from build123d import *

# Parameters (mm, degrees)
BOSS_EXTRUDE1_DEPTH = 12.7
SKETCH2_W           = 330.2
SKETCH2_H           = 19.05
CUT_EXTRUDE1_DEPTH  = 13.7
SKETCH3_R           = 1.27
CUT_EXTRUDE2_DEPTH  = 356.6
CUT_EXTRUDE7_DEPTH  = 6.35


with BuildPart() as part:
    # Sketch1 → Boss-Extrude1 (new body)
    with BuildSketch(Plane.XY):
        Polygon((0, 0), (355.6, 0), (355.6, -223.774), (274.574, -304.751813258), (81.026, -304.751813258), (0, -223.774), align=None)
    extrude(amount=BOSS_EXTRUDE1_DEPTH)

    # Sketch2 → Cut-Extrude1 (cut, through all)
    with BuildSketch(Plane.XY.offset(12.7)):
        with Locations((177.8, -9.525)):
            Rectangle(SKETCH2_W, SKETCH2_H)
    extrude(amount=-CUT_EXTRUDE1_DEPTH, mode=Mode.SUBTRACT)

    # Sketch3 → Cut-Extrude2 (cut, through all)
    with BuildSketch(Plane.ZY):
        with Locations((6.35, -6.35)):
            Circle(SKETCH3_R)
    extrude(amount=-CUT_EXTRUDE2_DEPTH, mode=Mode.SUBTRACT)

    # Sketch4 → Cut-Extrude7 (cut)
    with BuildSketch(Plane.XY):
        Polygon((10.3378, -45.974), (10.3378, -219.490141692), (85.306255844, -294.414013258), (86.209906071, -292.23149061), (12.520322648, -218.58573091), (12.520322648, -45.974), align=None)
        Polygon((270.293744156, -294.414013258), (345.2622, -219.490141692), (345.2622, -45.974), (342.9, -45.974), (342.9, -218.511274805), (269.416328936, -292.294854171), align=None)
    extrude(amount=CUT_EXTRUDE7_DEPTH, mode=Mode.SUBTRACT)


solid = part.part
Part model, mm, in its own coordinate system. A direction names the side the tool comes from. Give positions to 0.01 mm unless a question says otherwise; leave off trailing zeros. Write each loop counter-clockwise with the first axis right and the second up, starting at its lowest first coordinate (ties: lowest second). Pieces come first, ordered by that corner, then holes.
1) Probe L1, parallel to X at y = -201, z = 5.25; L2, parallel to Z at x = 2, y = -6; L3, parallel to X at y = -12, z = 5.25. List the from-to ranges inside material, lowest first.
Resolved:
L1: x = 0 to 10.34, 12.52 to 342.9, 345.26 to 355.6
L2: z = 0 to 5.13, 7.57 to 12.7
L3: x = 0 to 12.7, 342.9 to 355.6
2) Cut at A-A on z = 10.25. Write the cut outline in (x, y), then the cut area to 3 significant figures.
Resolved:
outline: (0, -223.77) - (81.03, -304.75) - (274.57, -304.75) - (355.6, -223.77) - (355.6, 0) - (342.9, 0) - (342.9, -19.05) - (12.7, -19.05) - (12.7, 0) - (0, 0) - close
area: 95,500 mm2
3) Pin check, flat tips, straight feed: pin 1 (2 mm diameter, centred on x = 43, z = 2, fed in from -Y); pin 2 (3 mm diameter, centred on x = 309.5, z = 3.5, fed in from -Y); pin 3 (3 mm diameter, centred on y = -6.35, z = 6.35, fed in from +X); pin 4 (2 mm diameter, centred on x = 235, z = 10.5, fed in from +Y). Stop position of each tip, or through.
Resolved:
pin 1: stops at y = -267.75
pin 2: stops at y = -271.35
pin 3: stops at x = 355.6
pin 4: stops at y = -19.05
4) Two-plate mould, pull along X, no slides. Class faces 1 (the face through (175, -19.05, 6)), 2 (the face through (179, -304.752, 6)), 3 (the face through (0, -113, 6)), 4 (the face through (315.65, -263.7, 6.26)): released by +X, released by -X, zero draft, split by the parting line, or undercut.
Resolved:
face 1: undercut
face 2: zero draft
face 3: released by -X
face 4: released by +X
5) Cut at D-D on x = 52.5. Write the cut outline in (y, z).
Resolved:
outline: (-276.24, 0) - (-261.63, 0) - (-261.63, 6.35) - (-258.54, 6.35) - (-258.54, 0) - (-19.05, 0) - (-19.05, 12.7) - (-276.24, 12.7) - close
6) Cut at C-C on y = -276. Write the cut outline in (x, z).
Resolved:
outline: (52.26, 0) - (66.88, 0) - (66.88, 6.35) - (69.97, 6.35) - (69.97, 0) - (285.64, 0) - (285.64, 6.35) - (288.72, 6.35) - (288.72, 0) - (303.34, 0) - (303.34, 12.7) - (52.26, 12.7) - close
7) Which spindle directions (+Z, -Z, +X, -X, +Y, -Y) get a long thin tool onto all of the face, cutting with end or side? Do faces 5 (the face through (47.3, -256.43, 3.13)), 6 (the face through (342.9, -10, 6)), 7 (the face through (180, -150, 12.7)). Say none if no direction does.
Resolved:
face 5: -Z
face 6: +Z, -Z, +Y
face 7: +Z, +X, -X, +Y, -Y
8) Cut at B-B on x = 261.5. Write the cut outline in (y, z).
Resolved:
outline: (-304.75, 0) - (-19.05, 0) - (-19.05, 12.7) - (-304.75, 12.7) - close
